Input: part model. Units: mm. Frame: model coordinates. Coordinates: 2 decimals unless noted, no trailing zeros. Loops run counter-clockwise (first coordinate to the right, second up) from the corner with the lowest first, then second, coordinate; pieces in that order, holes last. Notation, with made-up numbers: (29.25, 87) - (44.25, 87) arc R19 ccw to (44.25, 93) - close; hole circle Ø7 at (0, -5). An arc over 180 degrees is marked (long way). Use one line per item in the form item = value.
from build123d import *

# Parameters (mm, degrees)
BOSS_EXTRUDE1_DEPTH = 19.05
HOLE2_D             = 3.175
HOLE2_DEPTH         = 31.75
HOLE2_CSINK_D       = 10.16
HOLE2_CSINK_ANGLE   = 82
HOLE2_TIP           = 0.953866233
HOLE3_D             = 3.175
HOLE3_DEPTH         = 38.1
HOLE3_CSINK_D       = 10.16
HOLE3_CSINK_ANGLE   = 82
HOLE3_TIP           = 0.953866233


with BuildPart() as part:
    # Sketch1 → Boss-Extrude1 (new body)
    with BuildSketch(Plane.XY):
        with BuildLine():
            Line((-45.645654956, -462.283590669), (-43.591869521, -546.396382838))
            Line((-43.591869521, -546.396382838), (131.845939781, -542.11271078))
            Line((131.845939781, -542.11271078), (304.502022379, -82.799914861))
            Line((304.502022379, -82.799914861), (288.249001778, -54.142860136))
            Line((288.249001778, -54.142860136), (175.093421906, -22.889613201))
            Line((175.093421906, -22.889613201), (61.177817241, -435.332721236))
            ThreePointArc((61.177817241, -435.332721236), (69.660650717, -459.60790015), (43.950640658, -460.09591431))
            Line((43.950640658, -460.09591431), (-45.645654956, -462.283590669))
        make_face()
    extrude(amount=BOSS_EXTRUDE1_DEPTH)

    # Hole2
    with Locations(Plane(origin=(162.245907498, -21.702082459, 165.474999994), x_dir=(0, 0, -1), z_dir=(-0.9639097761610324, 0.2662291182819574, 0))):
        with Locations((-155.949999994, 107.734820482), (155.949999994, 107.734820482), (155.949999994, 327.755881328), (174.999999994, 85.732714397), (174.999999994, 349.757987412), (-174.999999994, 349.757987412), (-174.999999994, 85.732714397), (-155.949999994, 327.755881328)):
            CounterSinkHole(HOLE2_D / 2, HOLE2_CSINK_D / 2, depth=HOLE2_DEPTH, counter_sink_angle=HOLE2_CSINK_ANGLE)
            with Locations((0, 0, -(HOLE2_DEPTH + HOLE2_TIP / 2))):  # 118° drill point
                Cone(0, HOLE2_D / 2, HOLE2_TIP, mode=Mode.SUBTRACT)

    # Hole3
    with Locations(Plane(origin=(311.92831292, -63.043933951, -19.05), x_dir=(-0.3518626346959965, -0.9360516472421764, 8.51430303154421e-15), z_dir=(0, 0, -1))):
        with Locations((46.221112845, 113.488854888), (39.39759596, 37.945520226), (412.28786892, 80.423559293), (407.308516105, 25.297013484), (513.561319184, 161.164706775), (597.46020397, 127.267357003), (610.543339245, 159.649253123), (694.322923815, 367.011001477), (526.644454459, 193.546602895), (610.424039029, 400.908351249)):
            CounterSinkHole(HOLE3_D / 2, HOLE3_CSINK_D / 2, depth=HOLE3_DEPTH, counter_sink_angle=HOLE3_CSINK_ANGLE)
            with Locations((0, 0, -(HOLE3_DEPTH + HOLE3_TIP / 2))):  # 118° drill point
                Cone(0, HOLE3_D / 2, HOLE3_TIP, mode=Mode.SUBTRACT)


solid = part.part
Q1. Cut plane C-C, the plane x = 33. Return loops of the section in (y, z).
Check values:
outline = (-544.53, 0) - (-460.36, 0) - (-460.36, 19.05) - (-544.53, 19.05) - close
Q2. Pull-direction query (X, two-part tool) for faces 1 (the flat face through (166, -281, 19.05)), 2 (the cylindrical face through (69.896, -459.26, 9.392)), 3 (the flat face through (216.965, -315.672, 9.392)); classes: pulls with the +X half, pulls with the -X half, needs draft (parallel to the pull), parting line crosses it, or undercut.
Check values:
face_1 = needs draft
face_2 = undercut
face_3 = pulls with the +X half
Q3. Cut plane B-B, the plane y = -148.5. Return loops of the section in (x, z).
Check values:
outline = (140.4, 0) - (279.81, 0) - (279.81, 19.05) - (140.4, 19.05) - close
Q4. Cut plane A-A, the plane z = 16. Give the number of separate pieces and of enclosed holes in the cut face, then the cut area to 3 significant figures.
Check values:
separate_pieces = 1
enclosed_holes = 5
area = 69,300 mm²
Q5. Ray query, line 1 along Y through (x, z) = (-20.5, 6.75); line 2 along X through (y, z) = (-335.5, 9.5); line 3 along Y through (x, z) = (57, 11.5). Return the intervals inside material, ascending. Write a range as [from, to].
Check values:
line_1 = [-545.83, -488.39], [-485.73, -461.67]
line_2 = [88.75, 209.51]
line_3 = [-543.94, -466.41]
Q6. First-contact query: P1, Ø3, axis at x = 64, z = 9, coming from the -Y side; P2, Ø6, axis at y = -223.5, z = 9, coming from the +X side; P3, Ø2, axis at y = -152, z = 6.5, coming from the -X side. Flat tips, straight axial feed; report the tip coordinate or a pass-through.
Check values:
P1 = -543.81
P2 = 252.74
P3 = 139.16
